Design review of the part built by this model. Coordinates are the model's own, in mm. Face numbers are marked on the shaded views. A direction names the side the tool comes from. Coordinates: 2 decimals unless noted, no trailing zeros. Loops run counter-clockwise (first coordinate to the right, second up) from the corner with the lowest first, then second, coordinate; pieces in that order, holes last. Notation, with made-up numbers: M 66.5,-2.5 L 97.5,-2.5 A21 ccw 97.5,8.5 Z; hole C -4,29 d10. An arc over 180 degrees is marked long. Answer as a JSON object with one key per item and string values. Group by question number.
1. Consider section B-B (z = 4.5). State the section outline as (x, y) points (3 decimals), then the cut area to 3 significant figures.
2. To check wall thickness, follow probe 1 along X at (y, z) = (10, 1.25); probe 2 along X at (y, z) = (8.2, 4.5); probe 3 along Y at (x, z) = (16.5, 3.25). State the ranges of each line that lie inside material, in increasing order.
3. Consider section D-D (y = 11.5). State the section outline as (x, z) points.
4. Draft analysis for pull direction Y (two halves, no side actions). For the marked faces 3, 4 and 5, state which applies: +Y half, -Y half, draft (parallel to the pull), parting line (faces both ways), or undercut.
5. Consider section C-C (x = 6.1). State the section outline as (y, z) points.
6. Insertion check: pin 1 (12 mm diameter, centred on x = 8.5, z = 5, fed in from +Y); pin 2 (3 mm diameter, centred on x = 15.5, z = 3, fed in from -Y); pin 3 (1 mm diameter, centred on x = 15, y = 6, fed in from -Z); pin 4 (1.5 mm diameter, centred on y = 12, z = 6, fed in from +X). Each pin has a flat end and moves straight along its axis. Give the tip position at first contact, or say it passes through.
7. Machinability: for the marked faces 1 and 2, which of the approach directions +Z, -Z, +X, -X, +Y, -Y give a long, thin tool a straight path to every point of the face, cutting with its end or side? Answer none if there is none.
8. Consider section A-A (y = 8.2). State the section outline as (x, z) points, then the cut area to 3 significant figures.
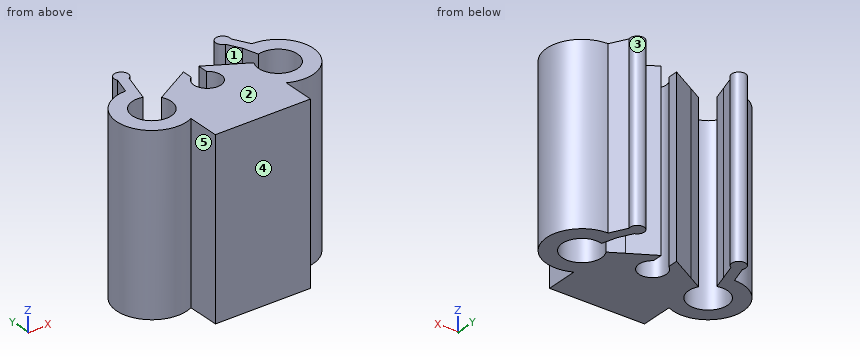
from build123d import *

# Parameters (mm, degrees)
Y_KSEKLIK_EKSTR_ZYON1_DEPTH = 22.43


with BuildPart() as part:
    # Çizim1 → Yükseklik-Ekstrüzyon1 (new body)
    with BuildSketch(Plane.XY):
        with BuildLine():
            ThreePointArc((5.113608786, 10.945521488), (6.1, 7.75), (7.086391214, 10.945521488))
            Line((7.086391214, 10.945521488), (7.086391214, 12.27879517))
            Line((7.086391214, 12.27879517), (10.2961903, 10.438363203))
            Line((10.2961903, 10.438363203), (12.031216834, 9.443535113))
            ThreePointArc((12.031216834, 9.443535113), (15.758549535, 6.245281773), (13.470670658, 10.591250449))
            Line((13.470670658, 10.591250449), (12.887207184, 12.504250808))
            Line((12.887207184, 12.504250808), (11.978588262, 14.203649507))
            ThreePointArc((11.978588262, 14.203649507), (11.817033945, 15.831345203), (13.080916647, 14.793032346))
            Line((13.080916647, 14.793032346), (14.2, 12.7))
            ThreePointArc((14.2, 12.7), (18.58121444, 7.172887527), (12.2, 4.168871126))
            Line((12.2, 4.168871126), (12.2, 0))
            Line((12.2, 0), (0, 0))
            Line((0, 0), (0, 4.168871126))
            ThreePointArc((0, 4.168871126), (-6.38121444, 7.172887527), (-2, 12.7))
            Line((-2, 12.7), (-1.311314062, 14.971308793))
            ThreePointArc((-1.311314062, 14.971308793), (-0.274595552, 16.23649961), (-0.115093584, 14.608601518))
            Line((-0.115093584, 14.608601518), (-0.747701793, 12.522238911))
            Line((-0.747701793, 12.522238911), (-1.304278774, 10.601243839))
            ThreePointArc((-1.304278774, 10.601243839), (-3.544803783, 6.234400531), (0.168783166, 9.443535113))
            Line((0.168783166, 9.443535113), (1.9038097, 10.438363203))
            Line((1.9038097, 10.438363203), (5.113608786, 12.27879517))
            Line((5.113608786, 12.27879517), (5.113608786, 10.945521488))
        make_face()
    extrude(amount=Y_KSEKLIK_EKSTR_ZYON1_DEPTH)


solid = part.part
Findings below:
{
 "1": {"outline": "M -2,12.7 A4.5 ccw long 0,4.169 L 0,0 L 12.2,0 L 12.2,4.169 A4.5 ccw long 14.2,12.7 L 13.081,14.793 A0.885 ccw long 11.979,14.204 L 12.887,12.504 L 13.471,10.591 A2.5 cw long 12.031,9.444 L 7.086,12.279 L 7.086,10.946 A1.75 cw long 5.114,10.946 L 5.114,12.279 L 0.169,9.444 A2.5 cw long -1.304,10.601 L -0.748,12.522 L -0.115,14.609 A0.885 ccw long -1.311,14.971 Z", "area": "188 mm^2"},
 "2": {"probe 1": "x = -6.12 to -3.73, 1.14 to 4.42, 7.78 to 11.06, 15.93 to 18.32", "probe 2": "x = -6.5 to -4.5, 0.5 to 4.93, 7.27 to 11.7, 16.7 to 18.7", "probe 3": "y = 4.33 to 7.22, 9.18 to 12.07"},
 "3": {"outline": "M -5.06,0 L -1.04,0 L -1.04,22.43 L -5.06,22.43 Z; M 3.76,0 L 5.11,0 L 5.11,22.43 L 3.76,22.43 Z; M 7.09,0 L 8.44,0 L 8.44,22.43 L 7.09,22.43 Z; M 13.19,0 L 17.26,0 L 17.26,22.43 L 13.19,22.43 Z"},
 "4": {"face 3": "undercut", "face 4": "-Y half", "face 5": "draft"},
 "5": {"outline": "M 0,0 L 7.75,0 L 7.75,22.43 L 0,22.43 Z"},
 "6": {"pin 1": "stops at y = 15.94", "pin 2": "stops at y = 3.7", "pin 3": "stops at z = 0", "pin 4": "stops at x = 17.51"},
 "7": {"face 1": "+Z, -Z", "face 2": "+Z, +X, -X, +Y, -Y"},
 "8": {"outline": "M -6.5,0 L -4.5,0 L -4.5,22.43 L -6.5,22.43 Z; M 0.5,0 L 4.93,0 L 4.93,22.43 L 0.5,22.43 Z; M 7.27,0 L 11.7,0 L 11.7,22.43 L 7.27,22.43 Z; M 16.7,0 L 18.7,0 L 18.7,22.43 L 16.7,22.43 Z", "area": "288 mm^2"}
}
